Could you check a few things on this drawing? It's one solid part, dimensions in mm from its lowest x, y, z. Coordinates: 2 decimals unless noted, no trailing zeros. Write each loop counter-clockwise with the first axis right and the second up, starting at its lowest first coordinate (ties: lowest second). Pieces come first, ordered by that corner, then holes. Notation, with made-up numbers: (-25, 71.25) - (-20, 71.25) arc R16 cw to (-20, 80.25) - close; hole circle Ø2 at (24.5, -18). An arc over 180 degrees is marked (long way). Answer as a JSON object with one key per item and string values. Group by question number.
1) If we section it at A-A (y = 5): Write out the boundary of the cut face in (x, z), plus the area to 3 significant figures.
2) If we section it at B-B (x = 32.5): Write out the boundary of the cut face in (y, z), plus the area to 3 significant figures.
3) Will these pins go through, and if not, where does the flat tip stop? pin 1 Ø3.5 at (y, z) = (4, 119) entering from +X; pin 2 Ø5 at (x, z) = (18.5, 83) entering from -Y; pin 3 Ø2 at (y, z) = (4, 3.5) entering from +X; pin 4 Ø2 at (x, y) = (36, 3) entering from +Z.
4) If we section it at C-C (z = 80.5): Write out the boundary of the cut face in (x, y).
5) Please list where these lines run through material, in increasing order: line 1 along X through (y, z) = (2.5, 111.5); line 2 along Z through (x, y) = (25.5, 2); line 3 along X through (y, z) = (1.75, 127.5).
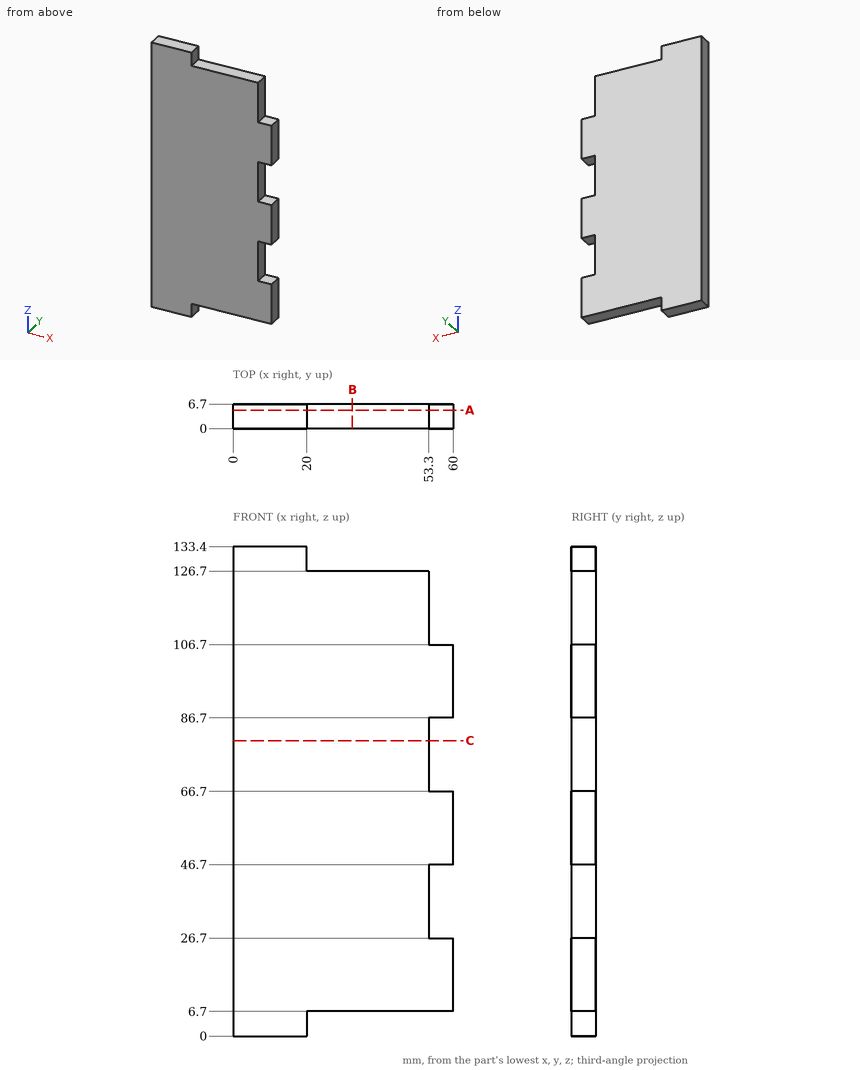
Here are the results:
{
 "1": {"outline": "(0, 0) - (20, 0) - (20, 6.7) - (60, 6.7) - (60, 26.7) - (53.3, 26.7) - (53.3, 46.7) - (60, 46.7) - (60, 66.7) - (53.3, 66.7) - (53.3, 86.7) - (60, 86.7) - (60, 106.7) - (53.3, 106.7) - (53.3, 126.7) - (20, 126.7) - (20, 133.4) - (0, 133.4) - close", "area": "7,070 mm²"},
 "2": {"outline": "(0, 6.7) - (6.7, 6.7) - (6.7, 126.7) - (0, 126.7) - close", "area": "804 mm²"},
 "3": {"pin 1": "stops at x = 53.3", "pin 2": "stops at y = 0", "pin 3": "stops at x = 20", "pin 4": "stops at z = 126.7"},
 "4": {"outline": "(0, 0) - (53.3, 0) - (53.3, 6.7) - (0, 6.7) - close"},
 "5": {"line 1": "x = 0 to 53.3", "line 2": "z = 6.7 to 126.7", "line 3": "x = 0 to 20"}
}
